Autodesk Inventor part; units mm, degrees
ref_plane "YZ Plane" through (0, 0, 0) normal (1, 0, 0) x (0, 1, 0)
ref_plane "XZ Plane" through (0, 0, 0) normal (0, 1, 0) x (-1, 0, 0)
ref_plane "XY Plane" through (0, 0, 0) normal (0, 0, 1) x (1, 0, 0)
sketch "Sketch1" plane through (0, 0, 0) normal (0, 1, 0) x (-1, 0, 0)
  circle A0 centre (0, 0) radius 35
  circle A1 centre (0, 0) radius 7.5
  dimension "d0" = 70
  dimension "d129" = 15
extrude "Extrusion1" add sketch "Sketch1" along normal blind 4
sketch "Sketch2" plane through (0, 4, 0) normal (0, 1, 0) x (1, 0, 0)
  circle A0 centre (0, 0) radius 30 construction
  point P0 (0, -30)
  point P1 (-25.9808, 15)
  point P2 (25.9808, 15)
  dimension "d130" = 60
  dimension "d131" = 120
  dimension "d132" = 120
hole "Hole1" at (-25.9808, 4, -15) at (25.9808, 4, -15) at (0, 4, 30) direction (0, -1, 0) diameter 3.2 end through all
sketch "Sketch16" plane through (0, 4, 0) normal (0, 1, 0) x (1, 0, 0)
  circle A0 centre (0, 0) radius 12 construction
  point P0 (0, -12)
  point P1 (-10.3923, 6)
  point P2 (10.3923, 6)
  dimension "d155" = 24
  dimension "d156" = 120
  dimension "d157" = 120
hole "Hole14" at (0, 4, 12) at (-10.3923, 4, -6) at (10.3923, 4, -6) direction (0, -1, 0) diameter 3.2 end through all
sketch "Sketch17" plane through (0, 4, 0) normal (0, 1, 0) x (1, 0, 0)
  circle A0 centre (0, 0) radius 12 construction
  point P0 (0, 12)
  point P1 (-10.3923, -6)
  point P2 (10.3923, -6)
  dimension "d165" = 24
  dimension "d166" = 120
  dimension "d167" = 120
hole "Hole15" at (0, 4, -12) at (-10.3923, 4, 6) at (10.3923, 4, 6) direction (0, -1, 0) diameter 2.459 end through all
sketch "Sketch18" plane through (0, 4, 0) normal (0, 1, 0) x (1, 0, 0)
  point P0 (0, 0)
  point P1 (20, 4.5)
  point P2 (20, -4.5)
  dimension "d175" = 9
  dimension "d176" = 4.5
  dimension "d177" = 20
hole "Hole16" at (20, 4, -4.5) at (20, 4, 4.5) direction (0, -1, 0) diameter 2.7 end through all
sketch "Sketch23" plane through (0, 4, 0) normal (0, 1, 0) x (1, 0, 0)
  point P0 (0, 0)
  point P1 (-20, 0)
  dimension "d238" = 20
hole "Hole21" at (-20, 4, 0) direction (0, -1, 0) diameter 3 end through all
sketch "Sketch24" plane through (0, 4, 0) normal (0, 1, 0) x (1, 0, 0)
  circle A0 centre (-20, 0) radius 1.5
  point P0 (0, 0)
  point P1 (-20, 6.1)
  point P2 (-20, -6.1)
  dimension "d246" = 12.2
  dimension "d247" = 6.1
hole "Hole22" at (-20, 4, -6.1) at (-20, 4, 6.1) direction (0, -1, 0) diameter 2.013 end through all
pattern_circular "Circular Pattern6" count 3 over 360 about axis through (0, 0, 0) along (0, 1, 0) of "Hole21", "Hole22"
pattern_circular "Circular Pattern7" count 3 over 360 about axis through (0, 0, 0) along (0, 1, 0) of "Hole16"
sketch "Sketch25" plane through (0, 4, 0) normal (0, 1, 0) x (1, 0, 0)
  circle A0 centre (0, 0) radius 30 construction
  circle A1 centre (0, -30) radius 1.6
  point P0 (12.2021, -27.4064)
  point P1 (22.2943, -20.0739)
  point P2 (28.5317, -9.2705)
  point P3 (29.8357, 3.1359)
  dimension "d261" = 60
  dimension "d262" = 24
  dimension "d263" = 24
  dimension "d264" = 24
  dimension "d275" = 24
hole "Hole23" at (12.2021, 4, 27.4064) at (22.2943, 4, 20.0739) at (28.5317, 4, 9.2705) at (29.8357, 4, -3.1359) direction (0, -1, 0) diameter 7 end through all
pattern_circular "Circular Pattern8" count 3 over 360 about axis through (0, 0, 0) along (0, 1, 0) of "Hole23"
properties part number "torsosc-frame-plate-v2" material "Copper"
The listing builds one solid part. Answer for the finished solid, in the listing's coordinates (mm). Round coordinates to 2 decimals unless told otherwise and drop trailing zeros. Write each loop counter-clockwise with the first axis right and the second up, starting at its lowest first coordinate (ties: lowest second). Pieces come first, ordered by that corner, then holes. Notation, with made-up numbers: M 6.25,5 L 34.25,5 A38 ccw 34.25,44 Z; hole C 77.5,27.25 d3. An arc over 180 degrees is marked long. Write each question's results on one line, items separated by ' | '. Start each with the question number.
Item 1: A cutting plane is placed at B-B on z = 30. Write down the section's boundary in (x, y), and give its area (3 significant figures).
Item 2: Flat-ended cylindrical pins translate along their axes: pin 1 Ø9 at (x, z) = (17.63, -24.27) entering from +Y; pin 2 Ø1 at (x, y) = (-12.5, 2) entering from +Z; pin 3 Ø1.5 at (x, y) = (-22.5, 2.5) entering from -Z; pin 4 Ø1 at (x, y) = (8.5, 3.5) entering from -Z. Find the tip coordinate at first contact, or state that the pin passes through.
Item 3: For a pull along Z with two mould halves and no side action, classify faces 1 (the face through (-6.508, 1.972, -18.283)), 2 (the face through (16.265, 1.972, 14.052)), 3 (the face through (0, 4, 8)) as pulls with the +Z half, pulls with the -Z half, needs draft (parallel to the pull), parting line crosses it, or undercut.
Item 4: Straight lines are drawn through the part: L1, parallel to Z at x = 0, y = 2.45; L2, parallel to X at y = 3, z = -24; L3, parallel to Z at x = -10, y = 0.6. For each, find the intervals that lie inside material, in ascending order. Write a range as [from, to].
Item 5: A cutting plane is placed at A-A on x = 0. Write down the section's boundary in (y, z), and give its area (3 significant figures).
Check sheet entries:
1) outline: M -18.03,0 L -14.55,0 L -14.55,4 L -18.03,4 Z; M -9.85,0 L -1.6,0 L -1.6,4 L -9.85,4 Z; M 1.6,0 L 9.85,0 L 9.85,4 L 1.6,4 Z; M 14.55,0 L 18.03,0 L 18.03,4 L 14.55,4 Z | area: 93.8 mm²
2) pin 1: y = 4 | pin 2: z = 32.88 | pin 3: z = -27.42 | pin 4: z = -34.07
3) face 1: undercut | face 2: undercut | face 3: needs draft
4) L1: [-35, -13.23], [-10.77, -7.5], [7.5, 10.4], [13.6, 28.4], [31.6, 35] | L2: [-25.48, -21.12], [-14.14, 14.14], [21.12, 25.48] | L3: [-33.54, -7.55], [-4.45, 4.83], [7.17, 24.69], [30.13, 33.54]
5) outline: M 0,-35 L 4,-35 L 4,-13.23 L 0,-13.23 Z; M 0,-10.77 L 4,-10.77 L 4,-7.5 L 0,-7.5 Z; M 0,7.5 L 4,7.5 L 4,10.4 L 0,10.4 Z; M 0,13.6 L 4,13.6 L 4,28.4 L 0,28.4 Z; M 0,31.6 L 4,31.6 L 4,35 L 0,35 Z | area: 185 mm²
